The model under review builds one solid part; all positions refer to its coordinate system, in mm. A direction names the side the tool comes from. Round coordinates to 2 decimals unless told otherwise and drop trailing zeros. Write each question's results on one line, items separated by ' | '.
```python
from build123d import *

# Parameters (mm, degrees)
INNERWHEEL_START                            = -0.79375
INNERWHEEL_OUTLINE_R                        = 4.28625
INNERWHEEL_DEPTH                            = 4.7625
CONNECTIONINNEROUTER_REACH                  = 43.498
CONNECTIONINNEROUTER_END_RADIUS             = 24.60625
SKETCH3_W                                   = 1.5875
SKETCH3_H                                   = 4.7625
CONNECTIONINNEROUTER_DIRECTION_2_REACH      = 43.498
CONNECTIONINNEROUTER_DIRECTION_2_END_RADIUS = 4.28625
CIRCULARPATTERN_COUNT                       = 6
MOTORSUPPORTEXTRUDE_DEPTH                   = 8
MOTORSUPPORTCUT_START                       = -8
MOTORSUPPORTCUT_DEPTH                       = 8
TIREFILLET_R                                = 1.5875


# Read off the part's stored shape, not the designer's step: InnerWheel
with BuildPart() as part:
    # OuterWheelSketch → OuterWheel (revolve)
    with BuildSketch(Plane.XY, mode=Mode.PRIVATE) as outerwheel_sk:
        Polygon((-25.4, 0), (-26.9875, 0), (-26.9875, -0.79375), (-24.60625, -0.79375), (-24.60625, 3.96875), (-26.9875, 3.96875), (-26.9875, 3.175), (-25.4, 3.175), align=None)
    revolve(outerwheel_sk.sketch.rotate(Axis((0, -1.962659061, 0), (0, 1, 0)), 270), axis=Axis((0, -1.962659061, 0), (0, 1, 0)))



with BuildPart() as body_2:
    # InnerWheel outline → InnerWheel (new body)
    with BuildSketch(Plane(origin=(0, 0, 0), x_dir=(1, 0, 0), z_dir=(0, 1, 0)).offset(INNERWHEEL_START)):
        Circle(INNERWHEEL_OUTLINE_R)
    extrude(amount=INNERWHEEL_DEPTH)


with BuildPart() as part_1:
    add(part.part)

    add(body_2.part)  # ConnectionInnerOuter merges body 2
    # ConnectionInnerOuter: up to this cylinder (the profile starts inside it)
    connectioninnerouter_end = Plane(origin=(0, 1.5875, 0), z_dir=(0, -1, 0)) * Cylinder(CONNECTIONINNEROUTER_END_RADIUS, 137.2085, mode=Mode.PRIVATE)
    # Sketch3 → ConnectionInnerOuter (add, up to the surface)
    with BuildSketch(Plane(origin=(4.28625, 0, 0), x_dir=(0, 0, -1), z_dir=(1, 0, 0)), mode=Mode.PRIVATE) as connectioninnerouter_sk1:
        with Locations((0, 1.5875)):
            Rectangle(SKETCH3_W, SKETCH3_H)
    connectioninnerouter_tool1 = extrude(connectioninnerouter_sk1.sketch, amount=CONNECTIONINNEROUTER_REACH, mode=Mode.PRIVATE) & connectioninnerouter_end
    connectioninnerouter = connectioninnerouter_tool1.solids().sort_by_distance((4.28625, 1.5875, 0))[0]
    add(connectioninnerouter)

    # ConnectionInnerOuter direction 2: up to this cylinder (the profile starts outside it)
    connectioninnerouter_direction_2_end = Plane(origin=(0, 1.5875, 0), z_dir=(0, -1, 0)) * Cylinder(CONNECTIONINNEROUTER_DIRECTION_2_END_RADIUS, 96.5685, mode=Mode.PRIVATE)
    # Sketch3 → ConnectionInnerOuter direction 2 (add, up to the surface)
    with BuildSketch(Plane(origin=(4.28625, 0, 0), x_dir=(0, 0, -1), z_dir=(1, 0, 0)), mode=Mode.PRIVATE) as connectioninnerouter_direction_2_sk1:
        with Locations((0, 1.5875)):
            Rectangle(SKETCH3_W, SKETCH3_H)
    connectioninnerouter_direction_2_tool1 = extrude(connectioninnerouter_direction_2_sk1.sketch, amount=-CONNECTIONINNEROUTER_DIRECTION_2_REACH, mode=Mode.PRIVATE) - connectioninnerouter_direction_2_end
    connectioninnerouter_direction_2 = connectioninnerouter_direction_2_tool1.solids().sort_by_distance((4.28625, 1.5875, 0))[0] + connectioninnerouter_direction_2_tool1.solids().sort_by_distance((4.28625, 1.5875, 0))[1]
    add(connectioninnerouter_direction_2)
    connectioninnerouter = connectioninnerouter + connectioninnerouter_direction_2  # both directions under the feature's name, for the pattern or mirror that repeats it

    # CircularPattern: ConnectionInnerOuter ×6 about axis
    circularpattern_axis = Axis((0, 0, 0), (0, 1, 0))
    for i in range(1, CIRCULARPATTERN_COUNT):
        add(connectioninnerouter.rotate(circularpattern_axis, i * 360 / CIRCULARPATTERN_COUNT))

    # OuterMottorSupport → MotorSupportExtrude (add)
    with BuildSketch(Plane(origin=(0, -0.79375, 0), x_dir=(-1, 0, 0), z_dir=(0, -1, 0))):
        with BuildLine():
            Line((-2.369154279, -3.302), (2.369154279, -3.302))
            ThreePointArc((2.369154279, -3.302), (4.064, 0), (2.369154279, 3.302))
            Line((2.369154279, 3.302), (-2.369154279, 3.302))
            ThreePointArc((-2.369154279, 3.302), (-4.064, 0), (-2.369154279, -3.302))
        make_face()
    extrude(amount=-MOTORSUPPORTEXTRUDE_DEPTH)

    # InnerMotorSupport → MotorSupportCut (cut)
    with BuildSketch(Plane(origin=(0, -0.79375, 0), x_dir=(-1, 0, 0), z_dir=(0, -1, 0)).offset(MOTORSUPPORTCUT_START)):
        with BuildLine():
            Line((-1.917657947, 2.032), (1.917657947, 2.032))
            ThreePointArc((1.917657947, 2.032), (2.794, 0), (1.917657947, -2.032))
            Line((1.917657947, -2.032), (-1.917657947, -2.032))
            ThreePointArc((-1.917657947, -2.032), (-2.794, 0), (-1.917657947, 2.032))
        make_face()
    extrude(amount=MOTORSUPPORTCUT_DEPTH, mode=Mode.SUBTRACT)

    # TireFillet
    tirefillet_edges = [part_1.edges().sort_by_distance(p)[0] for p in [
        (0, 0, 25.4),
        (0, 3.175, 25.4),
    ]]
    fillet(tirefillet_edges, radius=TIREFILLET_R - 0.0001)  # a hair under: the kernel refuses the full size


solid = part_1.part
```
Q1. Insertion check: P1, Ø3, axis at x = -13.5, y = 5.5, coming from the -Z side; P2, Ø1.6, axis at x = -0.5, y = 5.5, coming from the -Z side; P3, Ø3, axis at x = 5.5, y = 3.5, coming from the +Z side; P4, Ø2.5, axis at x = 0.5, y = 6, coming from the +Z side. Each pin has a flat end and moves straight along its axis. Give the tip position at first contact, or say it passes through.
Evaluation:
P1: passes through | P2: stops at z = -3.3 | P3: stops at z = 26.69 | P4: stops at z = 3.3
Q2. For probe 1 along X at (y, z) = (3, 1); probe 2 along Z at (x, y) = (-9.5, 3.75); probe 3 along X at (y, z) = (1, -4.5), list the stretches that pass through material, from the lowest coordinate up.
Evaluation:
probe 1: x = -26.24 to -24.59, -4.17 to -2.61, 2.61 to 4.17, 24.59 to 26.24 | probe 2: z = -25.26 to -22.7, -18.04 to -14.87, -0.79 to 0.79, 14.87 to 18.04, 22.7 to 25.26 | probe 3: x = -25.11 to -24.19, -3.51 to -1.68, 1.68 to 3.51, 24.19 to 25.11
Q3. We need section A-A (x = 0). State how many separate pieces and enclosed holes the cut face has, plus the area to 3 significant figures.
Evaluation:
separate pieces: 4 | enclosed holes: 0 | area: 44.5 mm^2
Q4. Tool access review of faces 5 (the flat face through (0, 6, 3.302)), 6 (the flat face through (0, -0.794, -4)), 7 (the flat face through (6.443, 1.554, -12.746)): name each direction out of +Z, -Z, +X, -X, +Y, -Y from which nothing blocks a thin tool from reaching the whole face with its end or side.
Evaluation:
face 5: +Z, +X, -X, +Y | face 6: +Z, -Z, +X, -X, -Y | face 7: +Y, -Y
Q5. The part is to be moulded in two halves that separate along X. For faces 1 (the flat face through (0.1, 7.206, 2.2)), 2 (the cylindrical face through (-2.794, 3.262, -0.032)), 3 (the cylindrical face through (-4.064, 5.565, 0.054)), 4 (the flat face through (7.817, 1.554, -11.953)), say which applies: released by +X, released by -X, zero draft, split by the parting line, or undercut.
Evaluation:
face 1: zero draft | face 2: undercut | face 3: released by -X | face 4: undercut
